from build123d import *

# Parameters (mm, degrees)
CUT_EXTRUDE_4_DEPTH      = 4
PATTERN_CIRCULAR_1_COUNT = 3
CUT_EXTRUDE_7_DEPTH      = 86.143936954
CUT_EXTRUDE_7_DEPTH_BACK = 86.143936954
SKETCH_12_W              = 25
SKETCH_12_H              = 15
CUT_EXTRUDE_START        = -6
SKETCH_13_W              = 17
SKETCH_13_H              = 62.633188826
CUT_EXTRUDE_12_DEPTH     = 6
CHAMFER_2_SIZE           = 0.3
CHAMFER_2_SIZE2          = 0.519615242
SKETCH_14_W              = 2
SKETCH_14_H              = 10
SKETCH_16_W              = 3
SKETCH_16_H              = 60.736072742
CUT_EXTRUDE_14_DEPTH     = 3
CHAMFER_3_SIZE           = 1
CUT_EXTRUDE_13_REACH     = 102.772


with BuildPart() as part:
    # Эскиз1 → Повернуть1 (revolve)
    with BuildSketch(Plane(origin=(0, 0, 0), x_dir=(0, 0, -1), z_dir=(1, 0, 0)), mode=Mode.PRIVATE) as revolve_1_sk:
        Polygon((0, 24.5), (70.999933333, 24.5), (70.999933333, 25.5), (72.999933333, 25.5), (72.999933333, 24.6), (74.999933333, 24.6), (74.999933333, 27), (25, 27), (25, 28.5), (0, 28.5), align=None)
    revolve(revolve_1_sk.sketch.rotate(Axis((0, 0, 0), (0, 0, -1)), 90), axis=Axis((0, 0, 0), (0, 0, -1)))

    # Эскиз9 → Вырез-Вытянуть4 (cut)
    with BuildSketch(Plane(origin=(0, 0, -74.999933333), x_dir=(-1, 0, 0), z_dir=(0, 0, -1))):
        with BuildLine():
            ThreePointArc((24.6, 0), (24.594916073, -0.500103353), (24.579666393, -1))
            Line((24.579666393, -1), (26.981475126, -1))
            ThreePointArc((26.981475126, -1), (26.995368384, -0.500085785), (27, 0))
            ThreePointArc((27, 0), (23.128631913, 13.930771186), (12.624712159, 23.866642891))
            Line((12.624712159, 23.866642891), (11.423807793, 21.786615513))
            ThreePointArc((11.423807793, 21.786615513), (21.049770447, 12.730560245), (24.6, 0))
        make_face()
    cut_extrude_4 = extrude(amount=-CUT_EXTRUDE_4_DEPTH, mode=Mode.SUBTRACT)

    # Круговой массив1: Вырез-Вытянуть4 ×3 about axis
    pattern_circular_1_axis = Axis((0, 0, 0), (0, 0, 1))
    for i in range(1, PATTERN_CIRCULAR_1_COUNT):
        add(cut_extrude_4.rotate(pattern_circular_1_axis, i * 360 / PATTERN_CIRCULAR_1_COUNT), mode=Mode.SUBTRACT)

    # Эскиз12 → Вырез-Вытянуть7 (cut, two sides: drawn at the far end of the back side and taken through both)
    with BuildSketch(Plane(origin=(0, 0, 0), x_dir=(1, 0, 0), z_dir=(0, 1, 0)).offset(-CUT_EXTRUDE_7_DEPTH_BACK)):
        with Locations((0, 13.5)):
            Rectangle(SKETCH_12_W, SKETCH_12_H)
    extrude(amount=CUT_EXTRUDE_7_DEPTH + CUT_EXTRUDE_7_DEPTH_BACK, mode=Mode.SUBTRACT)

    # Эскиз13 → Вырез-Вытянуть12 (cut)
    with BuildSketch(Plane.XY.offset(CUT_EXTRUDE_START)):
        Rectangle(SKETCH_13_W, SKETCH_13_H)
    extrude(amount=CUT_EXTRUDE_12_DEPTH, mode=Mode.SUBTRACT)

    # Фаска2
    chamfer_2_edges = [part.edges().sort_by_distance(p)[0] for p in [
        (-24.5, 0, -70.999933333),
    ]]
    chamfer_2_side = [part.faces().sort_by_distance(p)[0] for p in [
        (0, 24.746856587, -70.999933333),
    ]]
    chamfer(chamfer_2_edges, length=CHAMFER_2_SIZE, length2=CHAMFER_2_SIZE2, reference=chamfer_2_side[0])

    # Эскиз14 → Вырез-Повернуть1 (revolve, cut)
    with BuildSketch(Plane(origin=(0, 0, 0), x_dir=(0, 0, 1), z_dir=(-0.8986841034993474, -0.4385964912280702, 0))):
        with Locations((-21.5, -31.5)):
            Rectangle(SKETCH_14_W, SKETCH_14_H)
    revolve(axis=Axis((16.00877193, -32.801969778, -26.23783224), (0, 0, 1)), mode=Mode.SUBTRACT)

    # Эскиз16 → Вырез-Вытянуть14 (cut)
    with BuildSketch(Plane(origin=(-19.091883092, -19.091883092, 0), x_dir=(0, 0, 1), z_dir=(-0.7071067811865464, -0.7071067811865488, 0))):
        with Locations((-64.499933333, 0.711195231)):
            Rectangle(SKETCH_16_W, SKETCH_16_H)
    extrude(amount=-CUT_EXTRUDE_14_DEPTH, mode=Mode.SUBTRACT)

    # Фаска3
    # the kernel refuses this chamfer: 1 mm, written as the material it takes off along each edge
    with BuildSketch(Plane(origin=(-20.452659818, -13.488465679, -62.999933333), x_dir=(-0.5333586097594283, 0.8458892323439812, 0), z_dir=(0, 0, -1))) as chamfer_3_piece_1:
        with BuildLine():
            Line((1.002291345, 0), (CHAMFER_3_SIZE * 0.975275502088, -CHAMFER_3_SIZE * 0.220992522558))
            Line((CHAMFER_3_SIZE * 0.975275502088, -CHAMFER_3_SIZE * 0.220992522558), (0, 0))
            ThreePointArc((0, 0), (0.503575038, -0.005125864), (1.002291345, 0))
        make_face()
    extrude(amount=3, mode=Mode.SUBTRACT)
    with BuildSketch(Plane(origin=(-13.488465679, -20.452659818, -62.999933333), x_dir=(0.8458892323439845, -0.5333586097594231, 0), z_dir=(0, 0, -1))) as chamfer_3_piece_2:
        with BuildLine():
            Line((1.002291345, 0), (CHAMFER_3_SIZE * 0.975275502088, CHAMFER_3_SIZE * 0.220992522558))
            Line((CHAMFER_3_SIZE * 0.975275502088, CHAMFER_3_SIZE * 0.220992522558), (0, 0))
            ThreePointArc((0, 0), (0.503575038, 0.005125864), (1.002291345, 0))
        make_face()
    extrude(amount=3, mode=Mode.SUBTRACT)

    # Эскиз15 → Вырез-Вытянуть13 (cut, up to next)
    with BuildSketch(Plane(origin=(-19.091883092, -19.091883092, 0), x_dir=(0, 0, 1), z_dir=(-0.7071067811865464, -0.7071067811865488, 0)), mode=Mode.PRIVATE) as cut_extrude_13_sk1:
        with BuildLine():
            Line((-63, 6), (-63, -6))
            ThreePointArc((-63, -6), (-64.5, -7.5), (-66, -6))
            Line((-66, -6), (-66, 6))
            ThreePointArc((-66, 6), (-64.5, 7.5), (-63, 6))
        make_face()
    cut_extrude_13_tool1 = extrude(cut_extrude_13_sk1.sketch, amount=-CUT_EXTRUDE_13_REACH, mode=Mode.PRIVATE) & part.part
    add(cut_extrude_13_tool1.solids().sort_by_distance((-19.091883, -19.091883, -64.5))[0], mode=Mode.SUBTRACT)


solid = part.part
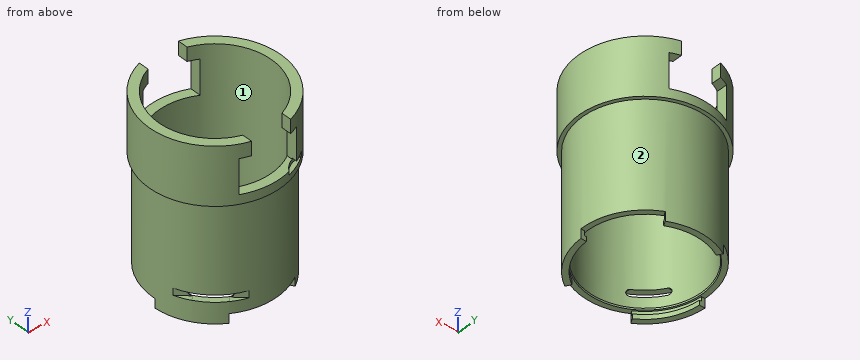
Model file for the job. Use its own axes, mm. Face numbers are marked on the shaded views. Give positions to 0.01 mm unless a question says otherwise; leave off trailing zeros. Order: outer loops, then holes, each group sorted by start corner. A loop starts at its lowest first (then second) coordinate and runs counter-clockwise, first axis right, second up. Notation, with made-up numbers: (62, -32.5) - (93, -32.5) arc R13 ccw to (93, -23.5) - close; hole circle Ø8 at (14, -33.75). An arc over 180 degrees is marked (long way). Return JSON: item names as keys, results as strings.
1) Flat gauge pins, fed straight in: P1, Ø3.5, axis at x = 21, y = -15, coming from the +Z side; P2, Ø1.5, axis at y = -17, z = -64, coming from the +X side; P3, Ø12, axis at x = 4, z = -18.5, coming from the +Y side; P4, Ø8, axis at x = -2.5, y = -24, coming from the +Z side. Where does each tip first touch, or does it go through?
Geometry says:
{"P1": "z = 0", "P2": "x = 21.56", "P3": "y = 28.5", "P4": "z = -21"}
2) Cut at D-D, the plane z = -51.5. Give the cut face in (x, y).
Geometry says:
{"outline": "circle Ø54 at (0, 0); hole circle Ø49 at (0, 0)"}
3) Probe line 1 (Y direction, x = 0, z = -43); line 2 (Z direction, x = -1, y = 26.5); line 3 (X direction, y = 12.5, z = -17). List the from-to ranges inside material, lowest first. Write a range as from..to.
Geometry says:
{"line 1": "-27..-24.5, 24.5..27", "line 2": "-75..-21", "line 3": "-25.61..-21.07, 21.07..25.61"}
4) Cut at B-B, the plane y = 0. Give the cut face in (x, z), plus the area to 3 significant figures.
Geometry says:
{"outline": "(-28.5, -25) - (-27, -25) - (-27, -71) - (-24.8, -71) - (-24.5, -70.48) - (-24.5, 0) - (-28.5, 0) - close; (24.5, -70.48) - (24.8, -71) - (27, -71) - (27, -25) - (28.5, -25) - (28.5, 0) - (24.5, 0) - close", "area": "430 mm²"}
5) Pull direction Y, two halves, no side cores. Call the marked faces 1 and 2: pulls with the +Y half, pulls with the -Y half, needs draft (parallel to the pull), parting line crosses it, or undercut.
Geometry says:
{"face 1": "undercut", "face 2": "parting line crosses it"}
6) Cut at C-C, the plane x = 0. Give the cut face in (y, z).
Geometry says:
{"outline": "(-28.5, -25) - (-27, -25) - (-27, -71) - (-24.8, -71) - (-24.5, -70.48) - (-24.5, -21) - (-28.5, -21) - close; (24.5, -70.48) - (24.8, -71) - (25.5, -71) - (25.5, -73) - (24.6, -73) - (24.6, -75) - (27, -75) - (27, -25) - (28.5, -25) - (28.5, -21) - (24.5, -21) - close"}
7) Cut at A-A, the plane z = -16. Give the cut face in (x, y), plus the area to 3 significant figures.
Geometry says:
{"outline": "(-12.5, -25.61) - (-12.5, -21.07) arc R24.5 cw to (-12.5, 21.07) - (-12.5, 25.61) arc R28.5 ccw to start; (12.5, -25.61) arc R28.5 ccw to (12.5, 25.61) - (12.5, 21.07) arc R24.5 cw to (12.5, -21.07) - close", "area": "458 mm²"}
